Autodesk Inventor part; units mm, degrees
ref_plane "YZ Plane" through (0, 0, 0) normal (1, 0, 0) x (0, 1, 0)
ref_plane "XZ Plane" through (0, 0, 0) normal (0, 1, 0) x (-1, 0, 0)
ref_plane "XY Plane" through (0, 0, 0) normal (0, 0, 1) x (1, 0, 0)
sketch "Sketch1" plane through (0, 0, 0) normal (0, 0, 1) x (1, 0, 0)
  circle A0 centre (0, 0) radius 12.7
  dimension "d0" = 25.4
extrude "Extrusion1" add sketch "Sketch1" along normal blind 6.35
sketch "Sketch2" plane through (0, 0, 0) normal (0, 0, -1) x (-1, 0, 0)
  point P0 (0, 0)
  point P1 (0, 0)
hole "Hole1" at (0, 0, 0) direction (0, 0, 1) diameter 8.4328 end through all
sketch "Sketch3" plane through (0, 0, 0) normal (0, 0, -1) x (-1, 0, 0)
  circle A0 centre (0, 0) radius 12.7
  circle A1 centre (0, 0) radius 12.7
  circle A2 centre (0, 0) radius 10.2864
  dimension "d10" = 20.5728
  dimension "d11" = 25.4
extrude "Extrusion2" add sketch "Sketch3" along normal blind 50.8
properties part number "topForDart"
Geometry: final body of the model. Coordinates: model frame, mm. Give positions to 0.01 mm unless a question says otherwise; leave off trailing zeros. Loops run counter-clockwise (first coordinate to the right, second up) from the corner with the lowest first, then second, coordinate; pieces in that order, holes last. Notation, with made-up numbers: (65.25, 5.5) -> (98.25, 5.5) arc R30 ccw to (98.25, 37.5) -> close; hole circle Ø11 at (17.25, 54.25). An arc over 180 degrees is marked (long way). Put each result on its own line as item: value.
1. Cut plane A-A (x = 0). Return the cut outline in (y, z), plus the area to 3 significant figures.
Taken from the geometry:
outline: (-12.7, -50.8) -> (-10.29, -50.8) -> (-10.29, 0) -> (-4.22, 0) -> (-4.22, 6.35) -> (-12.7, 6.35) -> close; (4.22, 0) -> (10.29, 0) -> (10.29, -50.8) -> (12.7, -50.8) -> (12.7, 6.35) -> (4.22, 6.35) -> close
area: 353 mm2
2. Cut plane D-D (y = 2.5). Return the cut outline in (x, z), plus the area to 3 significant figures.
Taken from the geometry:
outline: (-12.45, -50.8) -> (-9.98, -50.8) -> (-9.98, 0) -> (-3.4, 0) -> (-3.4, 6.35) -> (-12.45, 6.35) -> close; (3.4, 0) -> (9.98, 0) -> (9.98, -50.8) -> (12.45, -50.8) -> (12.45, 6.35) -> (3.4, 6.35) -> close
area: 366 mm2
3. Pull-direction query (Y, two-part tool) for faces 1 (the flat face through (4.4, 0.1, 0)), 2 (the cylindrical face through (2.23, 10.04, -25.04)), 3 (the flat face through (-4.64, -9.35, -50.8)); classes: released by +Y, released by -Y, zero draft, split by the parting line, or undercut.
Taken from the geometry:
face 1: undercut
face 2: undercut
face 3: zero draft
4. Cut plane B-B (z = -11). Return the cut outline in (x, y).
Taken from the geometry:
outline: circle Ø25.4 at (0, 0); hole circle Ø20.57 at (0, 0)
5. Pin query (flat end, axial travel): P1, Ø1.5, axis at x = -2, z = -24, coming from the -Y side; P2, Ø1, axis at x = 8, y = -5.5, coming from the -Z side; P3, Ø6, axis at x = 4, z = -6, coming from the -Y side. Return the tip coordinate at first contact, or that it passes through.
Taken from the geometry:
P1: stops at y = -12.64
P2: stops at z = 0
P3: stops at y = -12.66
6. Cut plane C-C (y = -7). Return the cut outline in (x, z), plus the area to 3 significant figures.
Taken from the geometry:
outline: (-10.6, -50.8) -> (-7.54, -50.8) -> (-7.54, 0) -> (7.54, 0) -> (7.54, -50.8) -> (10.6, -50.8) -> (10.6, 6.35) -> (-10.6, 6.35) -> close
area: 445 mm2
7. Ray query, line 1 along Y through (x, z) = (0, -14); line 2 along X through (y, z) = (0, 2.75). Return the intervals inside material, ascending. Write a range as [from, to].
Taken from the geometry:
line 1: y = [-12.7, -10.29], [10.29, 12.7]
line 2: x = [-12.7, -4.22], [4.22, 12.7]
